Geometry: final body of the model. Coordinates: model frame, mm. A direction names the side the tool comes from. Round coordinates to 2 decimals unless told otherwise and drop trailing zeros. Loops run counter-clockwise (first coordinate to the right, second up) from the corner with the lowest first, then second, coordinate; pieces in that order, holes last. Notation, with made-up numbers: M -25,74 L -19,74 A14 ccw -19,84 Z; hole C 8,-13 d5. An arc over 180 degrees is marked long. Answer as a JSON object with one key per item and string values.
from build123d import *

# Parameters (mm, degrees)
CROQUIS1_R                            = 6.1
SALIENTE_EXTRUIR1_DEPTH               = 20
CROQUIS3_R                            = 3
CORTAR_EXTRUIR1_DEPTH                 = 22.781184541
CROQUIS5_W                            = 1.3
CROQUIS5_H                            = 6.1
TALADRO_DE_MARGEN_PARA_M21_AT_2_COUNT = 2
TALADRO_DE_MARGEN_PARA_M21_AT_2_PITCH = 10


with BuildPart() as part:
    # Croquis1 → Saliente-Extruir1 (new body)
    with BuildSketch(Plane(origin=(0, 0, 0), x_dir=(-1, 0, 0), z_dir=(0, 1, 0))):
        with Locations(Location((0, 0, 0), (0, 0, 90))):
            Circle(CROQUIS1_R)
    extrude(amount=SALIENTE_EXTRUIR1_DEPTH)

    # Croquis3 → Cortar-Extruir1 (cut, through all)
    with BuildSketch(Plane.XZ):
        with Locations(Location((0, 0, 0), (0, 0, 270))):
            Circle(CROQUIS3_R)
    extrude(amount=-CORTAR_EXTRUIR1_DEPTH, mode=Mode.SUBTRACT)

    # Croquis5 → Taladro de margen para M21 (revolve, cut)
    with BuildSketch(Plane(origin=(0, 15, 0), x_dir=(0, -1, 0), z_dir=(1, 0, 0))):
        with Locations((0.65, 3.05)):
            Rectangle(CROQUIS5_W, CROQUIS5_H)
    taladro_de_margen_para_m21 = revolve(axis=Axis((0, 15, 6.35), (0, 0, -1)), mode=Mode.SUBTRACT)

    # Taladro de margen para M21 at 2: Taladro de margen para M21 ×2
    with Locations(*[(0, -i * TALADRO_DE_MARGEN_PARA_M21_AT_2_PITCH, 0) for i in range(1, TALADRO_DE_MARGEN_PARA_M21_AT_2_COUNT)]):
        add(taladro_de_margen_para_m21, mode=Mode.SUBTRACT)


solid = part.part
1) Reachability of faces 1 (the flat face through (3, 20, 1)), 2 (the cylindrical face through (-0.06, 6.3, -4.43)) from +Z, -Z, +X, -X, +Y, -Y: full face, straight path, thin tool, end or side. Return the list, or none.
Results:
{"face 1": "+Z, -Z, +X, -X, +Y", "face 2": "-Z"}
2) Section query D-D (y = 10.5). Return the cut outline in (x, z), and give its area (3 significant figures).
Results:
{"outline": "C 0,0 d12.2; hole C 0,0 d6", "area": "88.6 mm2"}
3) Ray query, line 1 (Y direction, x = 0, z = -5.15); line 2 (X direction, y = 6.5, z = 0); line 3 (X direction, y = 16.5, z = 1.75). Return the intervals inside material, ascending.
Results:
{"line 1": "0 to 3.7, 6.3 to 13.7, 16.3 to 20", "line 2": "-6.1 to -3, 3 to 6.1", "line 3": "-5.84 to -2.44, 2.44 to 5.84"}
4) Section query B-B (x = 0). Return the cut outline in (y, z).
Results:
{"outline": "M 0,-6.1 L 3.7,-6.1 L 3.7,-3 L 0,-3 Z; M 0,3 L 20,3 L 20,6.1 L 0,6.1 Z; M 6.3,-6.1 L 13.7,-6.1 L 13.7,-3 L 6.3,-3 Z; M 16.3,-6.1 L 20,-6.1 L 20,-3 L 16.3,-3 Z"}
5) Pin query (flat end, axial travel): P1, Ø2, axis at x = 3.5, y = 4.5, coming from the +Z side; P2, Ø4, axis at x = -3.5, y = 9, coming from the +Z side; P3, Ø1, axis at y = 17, z = 1, coming from the +X side. Return the tip coordinate at first contact, or that it passes through.
Results:
{"P1": "z = 5.56", "P2": "z = 5.91", "P3": "x = 6.08"}
6) Pull-direction query (X, two-part tool) for faces 3 (the cylindrical face through (1.83, 9.86, 5.82)), 4 (the cylindrical face through (0, 10, 3)), 5 (the flat face through (3, 0, 1)); classes: +X half, -X half, draft (parallel to the pull), parting line (faces both ways), or undercut.
Results:
{"face 3": "parting line", "face 4": "undercut", "face 5": "draft"}
7) Section query C-C (x = 2.5). Return the cut outline in (y, z), and give its area (3 significant figures).
Results:
{"outline": "M 0,-5.56 L 20,-5.56 L 20,-1.66 L 0,-1.66 Z; M 0,1.66 L 20,1.66 L 20,5.56 L 0,5.56 Z", "area": "156 mm2"}
8) Section query A-A (z = 0). Return the cut outline in (x, y).
Results:
{"outline": "M -6.1,0 L -3,0 L -3,20 L -6.1,20 Z; M 3,0 L 6.1,0 L 6.1,20 L 3,20 Z"}
